The listing builds one solid part. Answer for the finished solid, in the listing's coordinates (mm). Face numbers are marked on the shaded views. A direction names the side the tool comes from. Give positions to 0.01 mm unless a question says otherwise; leave off trailing zeros. Write each loop counter-clockwise with the first axis right and the second up, starting at its lowest first coordinate (ties: lowest second). Pieces come first, ordered by that corner, then holes.
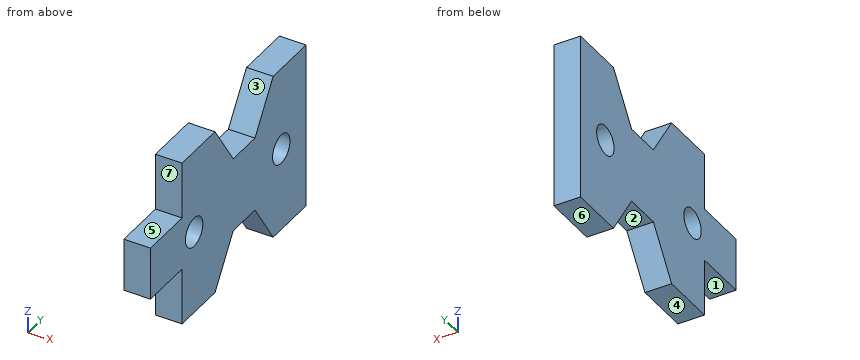
```python
from build123d import *

# Parameters (mm, degrees)
SKETCH1_R           = 1.75
BOSS_EXTRUDE1_DEPTH = 3.175


with BuildPart() as part:
    # Sketch1 → Boss-Extrude1 (new body)
    with BuildSketch(Plane(origin=(0, 0, 0), x_dir=(0, 0, -1), z_dir=(1, 0, 0))):
        Polygon((0, 0), (6.825, 0), (6.825, -6.35), (13.175, -6.35), (13.175, 0), (20, 0), (20, 6.629574014), (14.471500996, 10.288392178), (14.471500996, 14.663602622), (20, 18.322420786), (20, 24.9519948), (0, 24.9519948), (0, 18.322420786), (5.528499004, 14.663602622), (5.528499004, 10.288392178), (0, 6.629574014), align=None)
        with Locations((10, 19.9519948)):
            Circle(SKETCH1_R, mode=Mode.SUBTRACT)
        with Locations((10, 2.4259948)):
            Circle(SKETCH1_R, mode=Mode.SUBTRACT)
    extrude(amount=BOSS_EXTRUDE1_DEPTH)


solid = part.part
```
Item 1: Each of these flat-tipped pins is pushed along its axis until it touches: P1, Ø1.6, axis at x = 1, y = 12.5, coming from the -Z side; P2, Ø4.5, axis at y = 19.95, z = -10, coming from the +X side (3 decimals); P3, Ø1, axis at x = 2.5, y = 12.5, coming from the +Z side; P4, Ø1.6, axis at x = 2, y = -3.5, coming from the +Z side (3 decimals). Where does it stop, or does it pass through?
Conclusion:
P1: stops at z = -14.47
P2: stops at x = 3.175
P3: stops at z = -5.53
P4: stops at z = -6.825
Item 2: A cutting plane is placed at C-C, the plane z = -17.25. Give the vertices of the cut face in (x, y) (3 decimals).
Conclusion:
outline: (0, 0) - (3.175, 0) - (3.175, 8.45) - (0, 8.45) - close; (0, 16.502) - (3.175, 16.502) - (3.175, 24.952) - (0, 24.952) - close
Item 3: Determine the mould class of the marked faces 5, 6 and 7 for opening direction Z: pulls with the +Z half, pulls with the -Z half, needs draft (parallel to the pull), parting line crosses it, or undercut.
Conclusion:
face 5: pulls with the +Z half
face 6: pulls with the -Z half
face 7: needs draft
Item 4: A cutting plane is placed at B-B, the plane x = 2.65. Count the separate pieces of the cut face and the enclosed holes in it, plus the area to 3 significant figures.
Conclusion:
separate pieces: 1
enclosed holes: 2
area: 431 mm2
Item 5: Which of the six approach directions +Z, -Z, +X, -X, +Y, -Y give full straight-line access (tool end or side, diameter ignored) to the marked faces 1, 2, 3 and 4?
Conclusion:
face 1: -Z, +X, -X, -Y
face 2: -Z, +X, -X
face 3: +Z, +X, -X
face 4: -Z, +X, -X, +Y, -Y
Item 6: Consider probe 1 along Y at (x, z) = (1.75, -10); probe 2 along Y at (x, z) = (1.3, -11.25); probe 3 along Z at (x, y) = (2.3, -3.5) (3 decimals). Determine where each line is inside the solid, lowest interval first.
Conclusion:
probe 1: y = -6.35 to 0.68, 4.18 to 18.2, 21.7 to 24.95
probe 2: y = -6.35 to 1.2, 3.65 to 18.73, 21.18 to 24.95
probe 3: z = -13.175 to -6.825
Item 7: A cutting plane is placed at A-A, the plane z = -10. Give the vertices of the cut face in (x, y) (3 decimals).
Conclusion:
outline: (0, -6.35) - (3.175, -6.35) - (3.175, 0.676) - (0, 0.676) - close; (0, 4.176) - (3.175, 4.176) - (3.175, 18.202) - (0, 18.202) - close; (0, 21.702) - (3.175, 21.702) - (3.175, 24.952) - (0, 24.952) - close
Item 8: A cutting plane is placed at D-D, the plane y = -3.5. Give the vertices of the cut face in (x, z) (3 decimals).
Conclusion:
outline: (0, -13.175) - (3.175, -13.175) - (3.175, -6.825) - (0, -6.825) - close
